Verification items for the finished model (mm, model axes). Face numbers are marked on the shaded views. Give positions to 0.01 mm unless a question says otherwise; leave off trailing zeros. Order: outer loops, then holes, each group sorted by start corner. A loop starts at its lowest first (then second) coordinate and runs counter-clockwise, first axis right, second up.
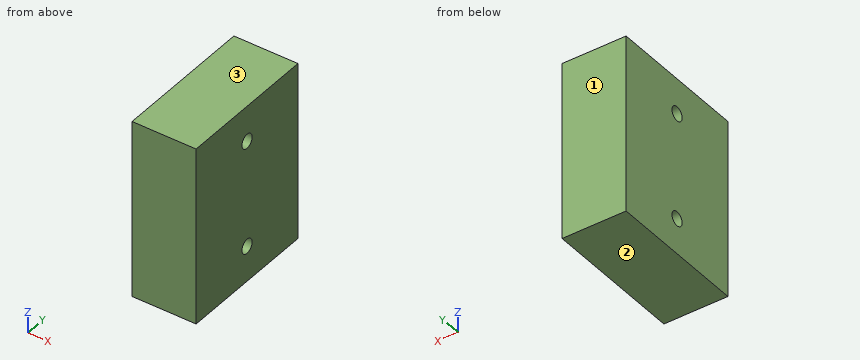
from build123d import *

# Parameters (mm, degrees)
CYLINDER028_R           = 2
CYLINDER028_DEPTH       = 20
CYLINDER028_PITCH_ANGLE = 90
ARRAY026_Z_COUNT        = 2
ARRAY026_Z_PITCH        = 30
BOX016_W                = 18
BOX016_H                = 40
BOX016_DEPTH            = 50


with BuildPart() as array026:
    # Cylinder028 → Cylinder028 (new body)
    with BuildSketch(Plane.XY):
        Circle(CYLINDER028_R)
    extrude(amount=CYLINDER028_DEPTH)


with BuildPart() as array026_1:
    # Cylinder028 pitch: moved
    add(array026.part.rotate(Axis((0, 0, 0), (0, 1, 0)), CYLINDER028_PITCH_ANGLE))


with BuildPart() as array026_2:
    # Cylinder028 placement: moved
    add(array026_1.part.moved(Location((134, 87, -14))))

    # Array026 Z: Array026 ×2


with BuildPart() as array026_3:
    add(array026_2.part)
    with Locations(*[(0, 0, -i * ARRAY026_Z_PITCH) for i in range(1, ARRAY026_Z_COUNT)]):
        add(array026_2.part)


with BuildPart() as case_2_con003:
    # Box016 → Box016 (new body)
    with BuildSketch(Plane(origin=(134, 67, -54), x_dir=(1, 0, 0), z_dir=(0, 0, 1))):
        with Locations((9, 20)):
            Rectangle(BOX016_W, BOX016_H)
    extrude(amount=BOX016_DEPTH)

    # Cut027: cut Array026
    add(array026_3.part, mode=Mode.SUBTRACT)


solid = case_2_con003.part
(1) Section check A-A, the plane y = 87. Enter the section's corners in (x, z).
Solved:
outline: (134, -54) - (152, -54) - (152, -46) - (134, -46) - close; (134, -42) - (152, -42) - (152, -16) - (134, -16) - close; (134, -12) - (152, -12) - (152, -4) - (134, -4) - close
(2) Release check for a two-part mould opening along Z. For the marked faces 1, 2 and 3 record: pulls with the +Z half, pulls with the -Z half, needs draft (parallel to the pull), parting line crosses it, or undercut.
Solved:
face 1: needs draft
face 2: pulls with the -Z half
face 3: pulls with the +Z half
(3) Scan lines: line 1 (Z direction, x = 140.75, y = 87); line 2 (Y direction, x = 142, z = -44); line 3 (Y direction, x = 142.75, z = -43). Record each from-to range of solid material in increasing order.
Solved:
line 1: z = -54 to -46, -42 to -16, -12 to -4
line 2: y = 67 to 85, 89 to 107
line 3: y = 67 to 85.27, 88.73 to 107
(4) Section check B-B, the plane z = -44. Enter the section's corners in (x, y), then the cut area to 3 significant figures.
Solved:
outline: (134, 67) - (152, 67) - (152, 85) - (134, 85) - close; (134, 89) - (152, 89) - (152, 107) - (134, 107) - close
area: 648 mm2
